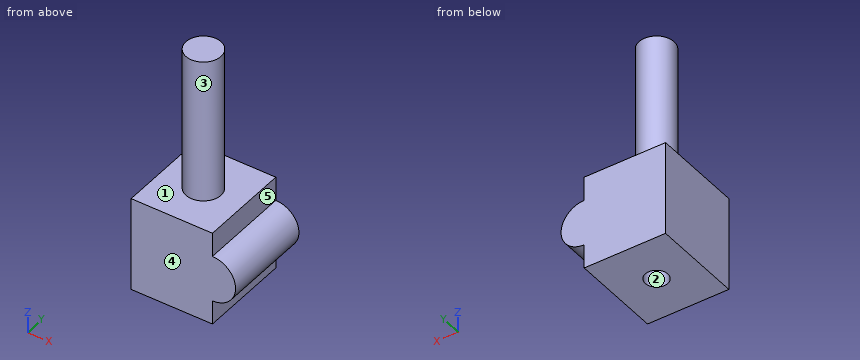
```python
from build123d import *

# Parameters (mm, degrees)
ESBO_O1_W                = 65
ESBO_O1_H                = 73
RESSALTO_EXTRUS_O1_DEPTH = 37.75
ESBO_O2_R                = 9
CORTE_EXTRUS_O1_DEPTH    = 105.5
ESBO_O3_R                = 14
RESSALTO_EXTRUS_O2_DEPTH = 115.5
ESBO_O4_R                = 18.5
RESSALTO_EXTRUS_O3_DEPTH = 73


with BuildPart() as part:
    # Esboço1 → Ressalto-extrusão1 (new body, symmetric)
    with BuildSketch(Plane.XY):
        Rectangle(ESBO_O1_W, ESBO_O1_H)
    extrude(amount=RESSALTO_EXTRUS_O1_DEPTH, both=True)

    # Esboço2 → Corte-extrusão1 (cut)
    with BuildSketch(Plane(origin=(0, 0, -37.75), x_dir=(-1, 0, 0), z_dir=(0, 0, -1))):
        Circle(ESBO_O2_R)
    extrude(amount=-CORTE_EXTRUS_O1_DEPTH, mode=Mode.SUBTRACT)

    # Esboço3 → Ressalto-extrusão2 (add)
    with BuildSketch(Plane.XY.offset(37.75)):
        Circle(ESBO_O3_R)
    extrude(amount=RESSALTO_EXTRUS_O2_DEPTH)

    # Esboço4 → Ressalto-extrusão3 (add)
    with BuildSketch(Plane(origin=(0, 36.5, 0), x_dir=(1, 0, 0), z_dir=(0, 1, 0))):
        with Locations((32.5, 0)):
            Circle(ESBO_O4_R)
    extrude(amount=-RESSALTO_EXTRUS_O3_DEPTH)


solid = part.part
```
For this review, take the finished solid that the model builds, in its own axes (mm). Face numbers are marked on the shaded views. A direction names the side the tool comes from. Coordinates: 2 decimals unless noted, no trailing zeros. Loops run counter-clockwise (first coordinate to the right, second up) from the corner with the lowest first, then second, coordinate; pieces in that order, holes last. Notation, with made-up numbers: (-18.5, -32.5) - (-3.5, -32.5) arc R29 ccw to (-3.5, 6.5) - close; hole circle Ø4 at (65.5, 54). An arc over 180 degrees is marked (long way). Use one line per item in the form item = value. Start each with the question number.
1) Take a section at A-A (x = 0). State the section outline as (y, z) points, plus the area to 3 significant figures.
2) Take a section at C-C (z = -16). State the section outline as (x, y) points, plus the area to 3 significant figures.
3) Draft analysis for pull direction Y (two halves, no side actions). For the marked faces 1, 2 and 3, state which applies: released by +Y, released by -Y, zero draft, split by the parting line, or undercut.
4) Take a section at D-D (y = -32). State the section outline as (x, z) points, plus the area to 3 significant figures.
5) Take a section at B-B (y = 0). State the section outline as (x, z) points, plus the area to 3 significant figures.
6) For the marked faces 4 and 5, list the 3-axis set-ups (+Z, -Z, +X, -X, +Y, -Y) from which the entire face can be reached by the end or side of a thin tool; tool diameter is ignored.
7) For pin 1 (4 mm diameter, centred on x = -17.5, y = 26, fed in from +Z); pin 2 (4 mm diameter, centred on x = 1, z = 89.5, fed in from -Y); pin 3 (6 mm diameter, centred on x = -14.5, z = 57.5, fed in from -Y), all flat-tipped, find the tip position at first contact; note any pin that passes through.
8) To check wall thickness, follow probe 1 along Y at (x, z) = (0, 7.5); probe 2 along Z at (x, y) = (2.5, 6.5); probe 3 along Z at (x, y) = (8, 28). State the ranges of each line that lie inside material, in increasing order. Write a range as from..to.
From the geometry:
q1.outline = (-36.5, -37.75) - (-9, -37.75) - (-9, 37.75) - (9, 37.75) - (9, -37.75) - (36.5, -37.75) - (36.5, 37.75) - (14, 37.75) - (14, 153.25) - (-14, 153.25) - (-14, 37.75) - (-36.5, 37.75) - close
q1.area = 7,390 mm2
q2.outline = (-32.5, -36.5) - (41.79, -36.5) - (41.79, 36.5) - (-32.5, 36.5) - close; hole circle Ø18 at (0, 0)
q2.area = 5,170 mm2
q3.face_1 = zero draft
q3.face_2 = undercut
q3.face_3 = split by the parting line
q4.outline = (-32.5, -37.75) - (32.5, -37.75) - (32.5, -18.5) arc R18.5 ccw to (32.5, 18.5) - (32.5, 37.75) - (-32.5, 37.75) - close
q4.area = 5,450 mm2
q5.outline = (-32.5, -37.75) - (-9, -37.75) - (-9, 37.75) - (9, 37.75) - (9, -37.75) - (32.5, -37.75) - (32.5, -18.5) arc R18.5 ccw to (32.5, 18.5) - (32.5, 37.75) - (14, 37.75) - (14, 153.25) - (-14, 153.25) - (-14, 37.75) - (-32.5, 37.75) - close
q5.area = 7,320 mm2
q6.face_4 = +Z, -Z, +X, -X, -Y
q6.face_5 = +Z, +X, +Y, -Y
q7.pin_1 = 37.75
q7.pin_2 = -14
q7.pin_3 = -7.98
q8.probe_1 = -36.5..-9, 9..36.5
q8.probe_2 = 37.75..153.25
q8.probe_3 = -37.75..37.75
